For this review, take the finished solid that the model builds, in its own axes (mm). A direction names the side the tool comes from. Give positions to 0.01 mm unless a question says otherwise; leave off trailing zeros. Loops run counter-clockwise (first coordinate to the right, second up) from the corner with the lowest first, then second, coordinate; pieces in that order, holes last.
```python
from build123d import *

# Parameters (mm, degrees)
F0_W     = 148.97
F0_H     = 123.57
F0_W_2   = 132.97
F0_H_2   = 107.57
F1_DEPTH = 4
F4_DEPTH = 10
F6_W     = 132.97
F6_H     = 107.57
F7_DEPTH = 4


# Not quite as in the source:
# - a pattern or mirror of a feature is missing from the dataset's text; its kind, count and spacing are read off the source's solid


with BuildPart() as f1:
    # F0 (on Top) → F1 (new body)
    with BuildSketch(Plane.XY):
        with Locations((70.485, -57.785)):
            Rectangle(F0_W, F0_H)
        with Locations((70.485, -57.785)):
            Rectangle(F0_W_2, F0_H_2, mode=Mode.SUBTRACT)
    extrude(amount=F1_DEPTH)

    # F2 (on face) → F4 (join)
    with BuildSketch(Plane(origin=(0, 0, 0), x_dir=(1, 0, 0), z_dir=(0, 0, -1))):
        Polygon((6, 119.57), (-4, 119.57), (-4, 109.57), (0, 109.57), (0, 115.57), (6, 115.57), align=None)
        Polygon((6, 0), (0, 0), (0, 6), (-4, 6), (-4, -4), (6, -4), align=None)
    f4 = extrude(amount=F4_DEPTH)

    # F4_copies: F4 across plane
    add(f4.mirror(Plane(origin=(70.485, 0, 0), x_dir=(0, 0, 1), z_dir=(1, 0, 0))))

    # F6 (on face) → F7 (join, through all)
    with BuildSketch(Plane.XY.offset(4)):
        with Locations((70.485, -57.785)):
            Rectangle(F6_W, F6_H)
    extrude(amount=-F7_DEPTH)


solid = f1.part
```
Q1. Consider section B-B on y = -24. Give the boundary of the cut face in (x, z).
Answers:
outline: (-4, 0) - (144.97, 0) - (144.97, 4) - (-4, 4) - close
Q2. Consider section C-C on x = 41. Give the boundary of the cut face in (y, z).
Answers:
outline: (-119.57, 0) - (4, 0) - (4, 4) - (-119.57, 4) - close
Q3. Mouldability with a two-part tool opening along X and no side actions: class faces 1 (the flat face through (0, -3, -5)), 2 (the flat face through (-2, -6, -5)), 3 (the flat face through (-4, -58.6, 0.2)) as +X half, -X half, draft (parallel to the pull), parting line (faces both ways), or undercut.
Answers:
face 1: undercut
face 2: draft
face 3: -X half
Q4. For pin 1 Ø6 at (y, z) = (-14.5, -5.5) entering from +X, flat-tipped, find the tip position at first contact; note if it passes through.
Answers:
pin 1: passes through
Q5. Consider section A-A on z = -7.25. Give the boundary of the cut face in (x, y).
Answers:
outline: (-4, -119.57) - (6, -119.57) - (6, -115.57) - (0, -115.57) - (0, -109.57) - (-4, -109.57) - close; (-4, -6) - (0, -6) - (0, 0) - (6, 0) - (6, 4) - (-4, 4) - close; (134.97, -119.57) - (144.97, -119.57) - (144.97, -109.57) - (140.97, -109.57) - (140.97, -115.57) - (134.97, -115.57) - close; (134.97, 0) - (140.97, 0) - (140.97, -6) - (144.97, -6) - (144.97, 4) - (134.97, 4) - close
Q6. Machinability: for faces 4 (the flat face through (144.97, -58.6, 0.2)), 5 (the flat face through (3, -115.57, -5)), 6 (the flat face through (143, -6, -5)), 7 (the flat face through (134.97, 2, -5)), which of the approach directions +Z, -Z, +X, -X, +Y, -Y give a long, thin tool a straight path to every point of the face, cutting with its end or side? Answer none if there is none.
Answers:
face 4: +Z, -Z, +X, +Y, -Y
face 5: -Z
face 6: -Z, +X, -X
face 7: -Z, +Y, -Y
Q7. For probe 1 along Z at (x, y) = (39.5, -72.5); probe 2 along X at (y, z) = (-3, -8.25), list the stretches that pass through material, from the lowest coordinate up.
Answers:
probe 1: z = 0 to 4
probe 2: x = -4 to 0, 140.97 to 144.97
